from build123d import *

# Parameters (mm, degrees)
EXTRUDE_1_DEPTH     = 4
SKETCH_3_R          = 1.55
CUT_EXTRUDE_1_DEPTH = 118.132745208
SHELL_1_T           = -2


with BuildPart() as part:
    # 草图1 → 凸台-拉伸1 (new body)
    with BuildSketch(Plane.XY):
        with BuildLine():
            Line((0.2, 40), (0.2, 18))
            ThreePointArc((0.2, 18), (1.020101013, 16.020101013), (3, 15.2))
            Line((3, 15.2), (6.5, 15.2))
            ThreePointArc((6.5, 15.2), (8.7627417, 14.2627417), (9.7, 12))
            Line((9.7, 12), (9.7, 3))
            ThreePointArc((9.7, 3), (10.520101013, 1.020101013), (12.5, 0.2))
            Line((12.5, 0.2), (89.5, 0.2))
            ThreePointArc((89.5, 0.2), (91.479898987, 1.020101013), (92.3, 3))
            Line((92.3, 3), (92.3, 12))
            ThreePointArc((92.3, 12), (93.2372583, 14.2627417), (95.5, 15.2))
            Line((95.5, 15.2), (99, 15.2))
            ThreePointArc((99, 15.2), (100.979898987, 16.020101013), (101.8, 18))
            Line((101.8, 18), (101.8, 40))
            ThreePointArc((101.8, 40), (100.979898987, 41.979898987), (99, 42.8))
            Line((99, 42.8), (95.5, 42.8))
            ThreePointArc((95.5, 42.8), (93.2372583, 43.7372583), (92.3, 46))
            Line((92.3, 46), (92.3, 55))
            ThreePointArc((92.3, 55), (91.479898987, 56.979898987), (89.5, 57.8))
            Line((89.5, 57.8), (12.5, 57.8))
            ThreePointArc((12.5, 57.8), (10.520101013, 56.979898987), (9.7, 55))
            Line((9.7, 55), (9.7, 46))
            ThreePointArc((9.7, 46), (8.7627417, 43.7372583), (6.5, 42.8))
            Line((6.5, 42.8), (3, 42.8))
            ThreePointArc((3, 42.8), (1.020101013, 41.979898987), (0.2, 40))
        make_face()
    extrude(amount=EXTRUDE_1_DEPTH)

    # 草图3 → 切除-拉伸1 (cut, through all)
    with BuildSketch(Plane.XY.offset(4)):
        with Locations((4, 39)):
            Circle(SKETCH_3_R)
        with Locations((4, 19)):
            Circle(SKETCH_3_R)
        with Locations((98, 39)):
            Circle(SKETCH_3_R)
        with Locations((98, 19)):
            Circle(SKETCH_3_R)
    extrude(amount=-CUT_EXTRUDE_1_DEPTH, mode=Mode.SUBTRACT)

    # 抽壳1
    shell_1_openings = [part.faces().sort_by_distance(p)[0] for p in [
        (51, 29, 0),
    ]]
    offset(amount=SHELL_1_T, openings=shell_1_openings, kind=Kind.INTERSECTION)


solid = part.part
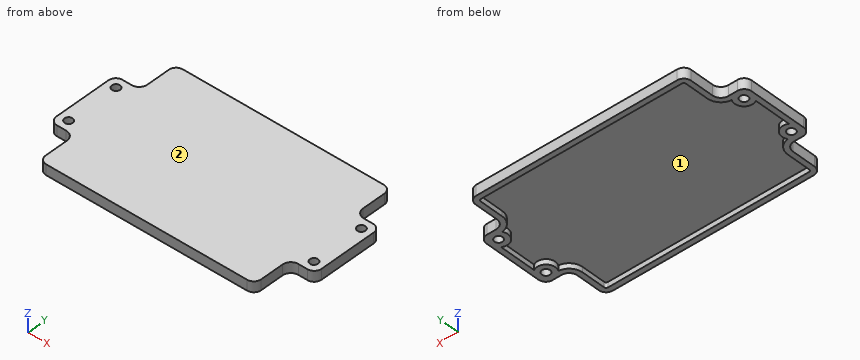
Part model, mm, in its own coordinate system. Face numbers are marked on the shaded views. Coordinates: 2 decimals unless noted, no trailing zeros. Write each loop counter-clockwise with the first axis right and the second up, starting at its lowest first coordinate (ties: lowest second). Pieces come first, ordered by that corner, then holes. Notation, with made-up numbers: (84.25, 37) - (107.25, 37) arc R14 ccw to (107.25, 58) - close; hole circle Ø3 at (-1, 10.25). An arc over 180 degrees is marked (long way). Put each result on its own line as item: value.
1. Band-saw the part on C-C (x = 56.5). Write the cut outline in (y, z), then the cut area to 3 significant figures.
Final values:
outline: (0.2, 0) - (2.2, 0) - (2.2, 2) - (55.8, 2) - (55.8, 0) - (57.8, 0) - (57.8, 4) - (0.2, 4) - close
area: 123 mm²
2. Flat gauge pins, fed straight in: pin 1 Ø2 at (y, z) = (48.5, 1) entering from +X; pin 2 Ø1.2 at (y, z) = (7.5, 1) entering from -X. Where does each tip first touch, or does it go through?
Final values:
pin 1: stops at x = 92.3
pin 2: stops at x = 9.7
3. Probe line 1 along Y through (x, z) = (98, 1.15); line 2 along Y through (x, z) = (98, 2.3); line 3 along Y through (x, z) = (71.5, 1.35). List the from-to ranges inside material, lowest first. Write a range as [from, to].
Final values:
line 1: y = [15.2, 17.45], [20.55, 22.55], [35.45, 37.45], [40.55, 42.8]
line 2: y = [15.2, 17.45], [20.55, 37.45], [40.55, 42.8]
line 3: y = [0.2, 2.2], [55.8, 57.8]
4. Band-saw the part on A-A (y = 19). Write the cut outline in (x, z).
Final values:
outline: (0.2, 0) - (2.45, 0) - (2.45, 4) - (0.2, 4) - close; (5.55, 0) - (7.55, 0) - (7.55, 2) - (94.45, 2) - (94.45, 0) - (96.45, 0) - (96.45, 4) - (5.55, 4) - close; (99.55, 0) - (101.8, 0) - (101.8, 4) - (99.55, 4) - close
5. Band-saw the part on B-B (x = 4). Write the cut outline in (y, z), then the cut area to 3 significant figures.
Final values:
outline: (15.2, 0) - (17.45, 0) - (17.45, 4) - (15.2, 4) - close; (20.55, 0) - (22.55, 0) - (22.55, 2) - (35.45, 2) - (35.45, 0) - (37.45, 0) - (37.45, 4) - (20.55, 4) - close; (40.55, 0) - (42.8, 0) - (42.8, 4) - (40.55, 4) - close
area: 59.8 mm²
6. Band-saw the part on D-D (y = 8). Write the cut outline in (x, z), then the cut area to 3 significant figures.
Final values:
outline: (9.7, 0) - (11.7, 0) - (11.7, 2) - (90.3, 2) - (90.3, 0) - (92.3, 0) - (92.3, 4) - (9.7, 4) - close
area: 173 mm²
7. Two-plate mould, pull along X, no slides. Class the marked faces 1 and 2: +X half, -X half, draft (parallel to the pull), parting line (faces both ways), or undercut.
Final values:
face 1: undercut
face 2: draft
